from build123d import *

# Parameters (mm, degrees)
F1_DEPTH = 152.4
F2_DEPTH = 19.05
F0_R     = 44.45
F3_DEPTH = 127
F4_DEPTH = 107.95


with BuildPart() as f1:
    # F0 (on Front) → F1 (new body)
    with BuildSketch(Plane.XZ):
        Polygon((79.34329, -243.498236), (79.34329, -192.698236), (-38.13171, -192.698236), (-57.18171, -192.698236), (-174.65671, -192.698236), (-174.65671, -243.498236), align=None)
    extrude(amount=F1_DEPTH)

    # F0 (on Front) → F2 (join)
    with BuildSketch(Plane.XZ):
        with BuildLine():
            ThreePointArc((-57.18171, -103.690338), (-98.575122, -78.850381), (-110.540249, -32.082083))
            Line((-110.540249, -32.082083), (-174.65671, -192.698236))
            Line((-174.65671, -192.698236), (-57.18171, -192.698236))
            Line((-57.18171, -192.698236), (-57.18171, -103.690338))
        make_face()
        with BuildLine():
            ThreePointArc((15.226829, -32.082083), (15.688987, -36.48468), (15.84329, -40.908777))
            ThreePointArc((15.84329, -40.908777), (0.494549, -82.305712), (-38.13171, -103.690338))
            Line((-38.13171, -103.690338), (-38.13171, -192.698236))
            Line((-38.13171, -192.698236), (79.34329, -192.698236))
            Line((79.34329, -192.698236), (15.226829, -32.082083))
        make_face()
    extrude(amount=F2_DEPTH)

    # F0 (on Front) → F3 (join)
    with BuildSketch(Plane.XZ):
        with BuildLine():
            ThreePointArc((-38.13171, -103.690338), (0.494549, -82.305712), (15.84329, -40.908777))
            ThreePointArc((15.84329, -40.908777), (15.688987, -36.48468), (15.226829, -32.082083))
            ThreePointArc((15.226829, -32.082083), (-47.65671, 22.591223), (-110.540249, -32.082083))
            ThreePointArc((-110.540249, -32.082083), (-98.575122, -78.850381), (-57.18171, -103.690338))
            ThreePointArc((-57.18171, -103.690338), (-47.65671, -104.408777), (-38.13171, -103.690338))
        make_face()
        with Locations((-47.65671, -40.908777)):
            Circle(F0_R, mode=Mode.SUBTRACT)
    extrude(amount=F3_DEPTH)

    # F0 (on Front) → F4 (join)
    with BuildSketch(Plane.XZ):
        with BuildLine():
            Line((-38.13171, -192.698236), (-38.13171, -103.690338))
            ThreePointArc((-38.13171, -103.690338), (-47.65671, -104.408777), (-57.18171, -103.690338))
            Line((-57.18171, -103.690338), (-57.18171, -192.698236))
            Line((-57.18171, -192.698236), (-38.13171, -192.698236))
        make_face()
    extrude(amount=F4_DEPTH)


solid = f1.part
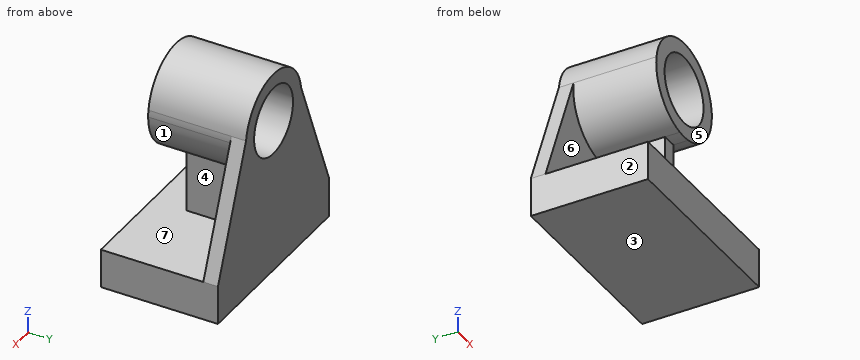
Work out the finished part from the listing and answer in its coordinate system (mm). Face numbers are marked on the shaded views. A direction names the side the tool comes from. Coordinates: 2 decimals unless noted, no trailing zeros. Loops run counter-clockwise (first coordinate to the right, second up) from the corner with the lowest first, then second, coordinate; pieces in that order, holes last. Notation, with made-up numbers: M -5,18.5 L 13,18.5 A14 cw 13,29.5 Z; hole C 64,55.5 d5. An arc over 180 degrees is marked long. Answer in a Markdown table with one row per item. Add a question column.
1. Find section B-B, the plane y = -42. Write down the section's boundary in (x, z), then the cut area to 3 significant figures.
2. The mould has two halves that part along Z. Classify the marked faces 1, 2 and 3: pulls with the +Z half, pulls with the -Z half, needs draft (parallel to the pull), parting line crosses it, or undercut.
3. Find section C-C, the plane z = -56.5. Write down the section's boundary in (x, y), then the cut area to 3 significant figures.
4. Find section A-A, the plane x = -61. Write down the section's boundary in (y, z), then the cut area to 3 significant figures.
5. A tool of negligible diameter and unlimited length cuts with its end or side. For the marked faces 4, 5, 6 and 7, from which of +Z, -Z, +X, -X, +Y, -Y can it reach the whole face along a straight path? Write none if from no direction.
6. Flat-ended cylindrical pins translate along their axes: P1, Ø2, axis at y = -116.5, z = -56.5, coming from the -X side; P2, Ø9.5, axis at x = -51.5, z = -159.5, coming from the -Y side; P3, Ø1.5, axis at x = 30, y = -105.5, coming from the +Z side. Find the tip coordinate at first contact, or state that the pin passes through.
7. Consider L1, parallel to Z at x = -93, y = -70.5; L2, parallel to Y at x = 22, z = -112.5; L3, parallel to X at y = -20.5, z = -31. Determine where each line is inside the solid, lowest interval first.
8. Find section D-D, the plane z = -109.5. Write down the section's boundary in (x, y).
Reported:
| question | item | result |
|---|---|---|
| 1 | outline | M -174.66,-243.5 L 79.34,-243.5 L 79.34,-192.7 L -38.13,-192.7 L -38.13,-103.69 A63.5 ccw 15.84,-40.91 A63.5 ccw 15.23,-32.08 A63.5 ccw long -57.18,-103.69 L -57.18,-192.7 L -174.66,-192.7 Z; hole C -47.66,-40.91 d88.9 |
| 1 | area | 21,100 mm^2 |
| 2 | face 1 | undercut |
| 2 | face 2 | needs draft |
| 2 | face 3 | pulls with the -Z half |
| 3 | outline | M -120.29,-19.05 L -109.21,-19.05 L -109.21,-127 L -89.28,-127 L -89.28,0 L -120.29,0 Z; M -6.03,-127 L 13.9,-127 L 13.9,-19.05 L 24.97,-19.05 L 24.97,0 L -6.03,0 Z |
| 3 | area | 5,480 mm^2 |
| 4 | outline | M -152.4,-243.5 L 0,-243.5 L 0,-83.31 L -127,-83.31 L -127,-102.99 L -19.05,-102.99 L -19.05,-192.7 L -152.4,-192.7 Z; M -127,1.49 L 0,1.49 L 0,21.17 L -127,21.17 Z |
| 4 | area | 14,500 mm^2 |
| 5 | face 4 | +X, -Y |
| 5 | face 5 | +Z, +X, -X, -Y |
| 5 | face 6 | -X, -Y |
| 5 | face 7 | -Y |
| 6 | P1 | stops at x = -109.46 |
| 6 | P2 | stops at y = -107.95 |
| 6 | P3 | stops at z = -192.7 |
| 7 | L1 | z = -243.5 to -192.7, -85.36 to 3.55 |
| 7 | L2 | y = -19.05 to 0 |
| 7 | L3 | x = -110.38 to -90.99, -4.33 to 15.07 |
| 8 | outline | M -141.44,-19.05 L -57.18,-19.05 L -57.18,-107.95 L -38.13,-107.95 L -38.13,-19.05 L 46.13,-19.05 L 46.13,0 L -141.44,0 Z |
